Could you check a few things on this drawing? It's one solid part, dimensions in mm from its lowest x, y, z. A direction names the side the tool comes from. Give positions to 0.01 mm unless a question says otherwise; leave off trailing zeros. Order: outer loops, then holes, each group sorted by start corner. A loop starts at its lowest first (then second) coordinate and runs counter-clockwise, first axis right, second up. Notation, with made-up numbers: (87, 21) - (103, 21) arc R34 ccw to (103, 54) - close; hole circle Ø4 at (80, -15.75). An arc over 180 degrees is marked (long way). Answer as CSV lines item,"result".
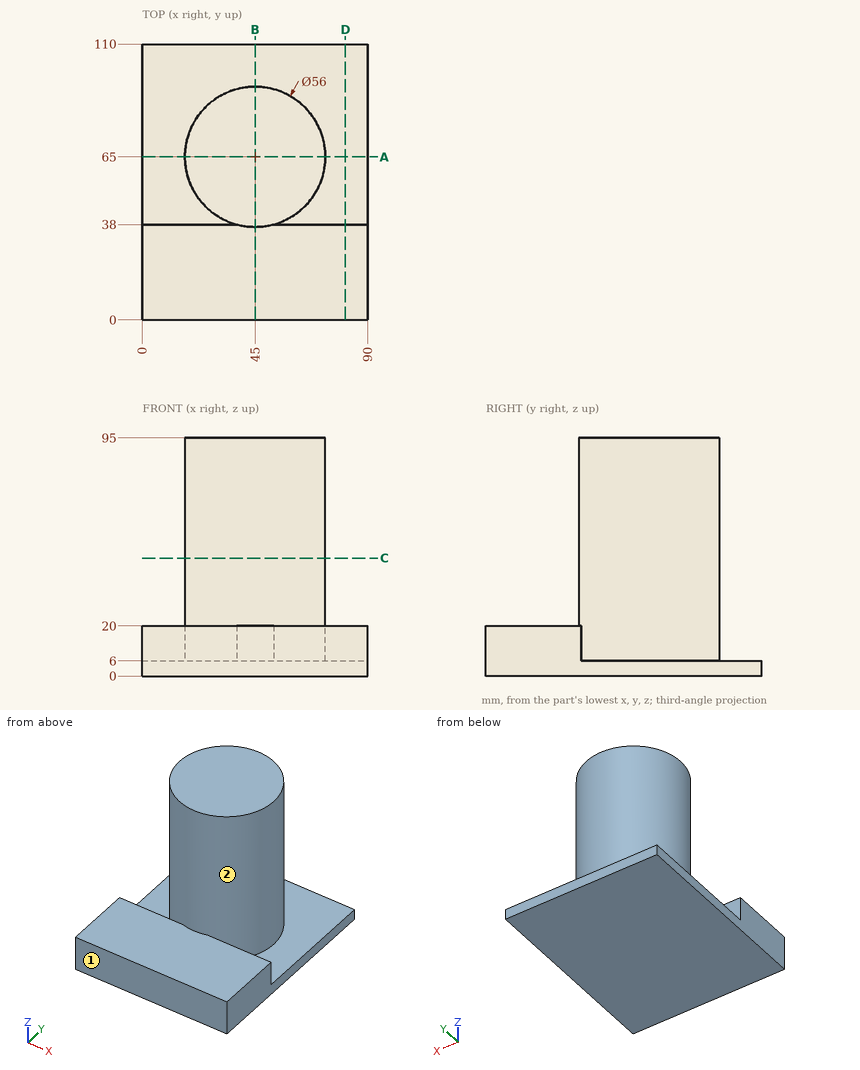
1) I need wall thicknesses on line 1 along Z through (x, y) = (7, 97); line 2 along Z through (x, y) = (29, 30); line 3 along Y through (x, z) = (28, 15). Which ranges of each line are inside material? Lowest first, please. Write a range as [from, to].
Answer block:
line 1,"[0, 6]"
line 2,"[0, 20]"
line 3,"[0, 38], [42.75, 87.25]"
2) I want a section at A-A on y = 65. Write out the boundary of the cut face in (x, z), plus the area to 3 significant figures.
Answer block:
outline,"(0, 0) - (90, 0) - (90, 6) - (73, 6) - (73, 95) - (17, 95) - (17, 6) - (0, 6) - close"
area,"5,520 mm2"
3) Which directions (+Z, -Z, +X, -X, +Y, -Y) give clear straight access to the entire face, cutting with the end or side of a thin tool? Please do the marked faces 1 and 2.
Answer block:
face 1,"+Z, -Z, +X, -X, -Y"
face 2,"+Z"
4) I'm going to push flat-ended pins straight in: P1, Ø2, axis at x = 64.5, z = 61.5, coming from the +Y side; P2, Ø10, axis at y = 46, z = 77.5, coming from the -X side; P3, Ø3, axis at y = 58, z = 18.5, coming from the -X side. Where does each tip first touch, or does it pass through?
Answer block:
P1,"y = 86.02"
P2,"x = 20.75"
P3,"x = 17.55"
5) I want a section at B-B on x = 45. Write out the boundary of the cut face in (y, z), plus the area to 3 significant figures.
Answer block:
outline,"(0, 0) - (110, 0) - (110, 6) - (93, 6) - (93, 95) - (37, 95) - (37, 20) - (0, 20) - close"
area,"6,160 mm2"
6) I want a section at C-C on z = 47. Write out the boundary of the cut face in (x, y).
Answer block:
outline,"circle Ø56 at (45, 65)"
7) I want a section at D-D on x = 81. Write out the boundary of the cut face in (y, z).
Answer block:
outline,"(0, 0) - (110, 0) - (110, 6) - (38, 6) - (38, 20) - (0, 20) - close"
